Design review of the part built by this model. Coordinates are the model's own, in mm. Coordinates: 2 decimals unless noted, no trailing zeros. Order: outer loops, then holes, each group sorted by start corner. A loop starts at its lowest first (then second) coordinate and runs counter-clockwise, first axis right, second up. Notation, with made-up numbers: (47, 46) -> (83, 46) arc R4 ccw to (83, 50) -> close; hole circle Ø1 at (8, 54.25). An arc over 180 degrees is marked (long way). Write item = value, one per line.
```python
from build123d import *

# Parameters (mm, degrees)
SKETCH_1_W          = 38
SKETCH_1_H          = 10
EXTRUDE_1_DEPTH     = 10
SKETCH_3_R          = 2
CUT_EXTRUDE_1_DEPTH = 10
SKETCH_4_R          = 2
CUT_EXTRUDE_2_DEPTH = 10


with BuildPart() as part:
    # 草图1 → 凸台-拉伸1 (new body)
    with BuildSketch(Plane.XY):
        Rectangle(SKETCH_1_W, SKETCH_1_H)
    extrude(amount=EXTRUDE_1_DEPTH)

    # 草图3 → 切除-拉伸1 (cut)
    with BuildSketch(Plane.XY.offset(10)):
        with Locations((-11, 0)):
            Circle(SKETCH_3_R)
        with Locations(Location((11, 0, 0), (0, 0, 180))):
            Circle(SKETCH_3_R)
    extrude(amount=-CUT_EXTRUDE_1_DEPTH, mode=Mode.SUBTRACT)

    # 草图4 → 切除-拉伸2 (cut)
    with BuildSketch(Plane(origin=(0, 5, 0), x_dir=(1, 0, 0), z_dir=(0, 1, 0))):
        with Locations(Location((-6, -5, 0), (0, 0, 270))):
            Circle(SKETCH_4_R)
        with Locations(Location((6, -5, 0), (0, 0, 90))):
            Circle(SKETCH_4_R)
    extrude(amount=-CUT_EXTRUDE_2_DEPTH, mode=Mode.SUBTRACT)


solid = part.part
```
(1) For L1, parallel to X at y = -2.25, z = 5; L2, parallel to Y at x = -11, z = 8; L3, parallel to Z at x = 6, y = 2.75, list the stretches that pass through material, from the lowest coordinate up.
Report:
L1 = -19 to -8, -4 to 4, 8 to 19
L2 = -5 to -2, 2 to 5
L3 = 0 to 3, 7 to 10
(2) We need section A-A (y = 0). Write out the cut boundary in (x, z), and give its area (3 significant figures).
Report:
outline = (-19, 0) -> (-13, 0) -> (-13, 10) -> (-19, 10) -> close; (-9, 0) -> (9, 0) -> (9, 10) -> (-9, 10) -> close; (13, 0) -> (19, 0) -> (19, 10) -> (13, 10) -> close; hole circle Ø4 at (-6, 5); hole circle Ø4 at (6, 5)
area = 275 mm²
(3) The part is to be moulded in two halves that separate along Z. For faces 1 (the cylindrical face through (7.2, 0.1, 6.6)), 2 (the flat face through (0, 0, 0)), 3 (the flat face through (0, 5, 5)), say which applies: released by +Z, released by -Z, zero draft, split by the parting line, or undercut.
Report:
face_1 = undercut
face_2 = released by -Z
face_3 = zero draft
(4) We need section B-B (z = 5). Write out the cut boundary in (x, y), and give its area (3 significant figures).
Report:
outline = (-19, -5) -> (-8, -5) -> (-8, 5) -> (-19, 5) -> close; (-4, -5) -> (4, -5) -> (4, 5) -> (-4, 5) -> close; (8, -5) -> (19, -5) -> (19, 5) -> (8, 5) -> close; hole circle Ø4 at (-11, 0); hole circle Ø4 at (11, 0)
area = 275 mm²
(5) We need section C-C (x = -6). Write out the cut boundary in (y, z).
Report:
outline = (-5, 0) -> (5, 0) -> (5, 3) -> (-5, 3) -> close; (-5, 7) -> (5, 7) -> (5, 10) -> (-5, 10) -> close
(6) Insertion check: pin 1 (3 mm diameter, centred on x = 6, z = 5, fed in from -Y). The pin has a flat end and moves straight along its axis. Give the tip position at first contact, or say it passes through.
Report:
pin_1 = through
(7) We need section D-D (y = -3.75). Write out the cut boundary in (x, z).
Report:
outline = (-19, 0) -> (19, 0) -> (19, 10) -> (-19, 10) -> close; hole circle Ø4 at (-6, 5); hole circle Ø4 at (6, 5)
